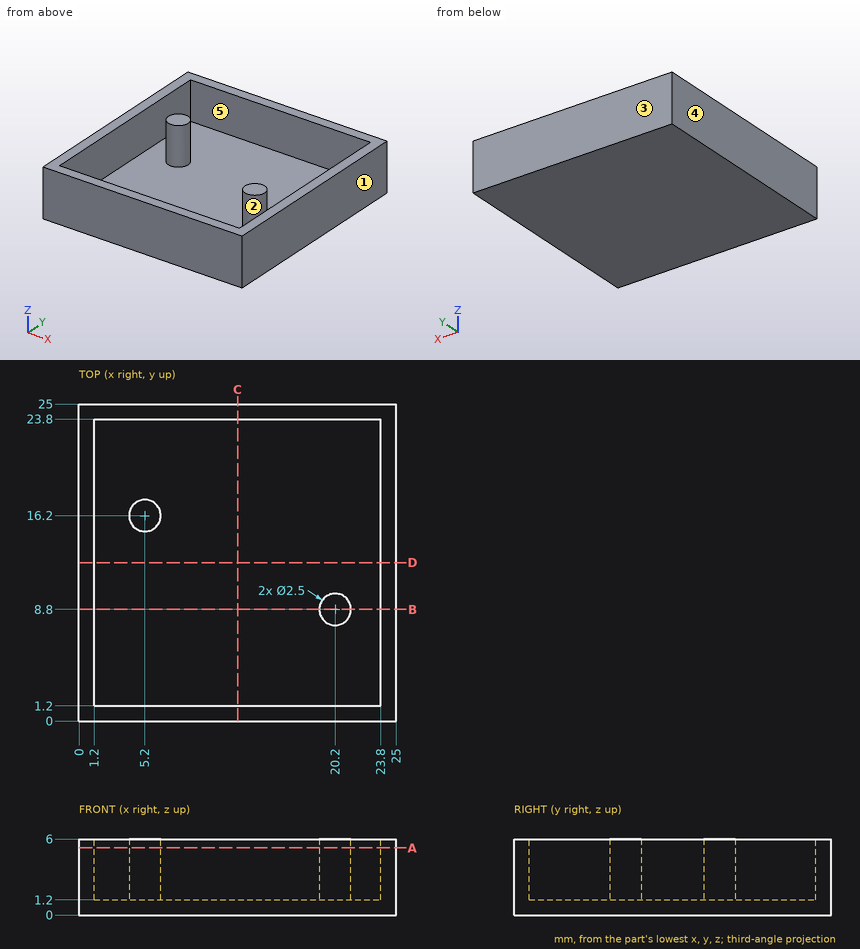
Geometry check sheet. Reference: drawing and pictorial views, mm from the part's lowest x, y, z. A direction names the side the tool comes from. Round coordinates to 2 decimals unless told otherwise and drop trailing zeros. Loops run counter-clockwise (first coordinate to the right, second up) from the corner with the lowest first, then second, coordinate; pieces in that order, holes last. Notation, with made-up numbers: (-30.5, -26.75) - (-1.5, -26.75) arc R13 cw to (-1.5, -5.75) - close; hole circle Ø3 at (9, -25). An arc over 180 degrees is marked (long way). Answer in a Markdown table with one row per item. Add a question column.
Q1. Section check A-A on z = 5.3. Enter the section's corners in (x, y), plus the area to 3 significant figures.
Q2. Section check B-B on y = 8.8. Enter the section's corners in (x, z).
Q3. Section check C-C on x = 12.5. Enter the section's corners in (y, z).
Q4. Gauge pin test, flat ends, axial feed: pin 1 (12 mm diameter, centred on x = 18, y = 13, fed in from -Z); pin 2 (1.5 mm diameter, centred on x = 9.5, y = 12, fed in from +Z). Record the tip position at first contact, or that the pin passes through.
Q5. Tool access check on the marked faces 4 and 5. Record the directions out of +Z, -Z, +X, -X, +Y, -Y that give a thin tool (end or side, any length) a straight path to the whole face; none if there is none.
Q6. Release check for a two-part mould opening along X. For the marked faces 1, 2 and 3 record: pulls with the +X half, pulls with the -X half, needs draft (parallel to the pull), parting line crosses it, or undercut.
Q7. Material ranges on line 1 (Y direction, x = 21.5, z = 1.75); line 2 (Y direction, x = 20.75, z = 1.5), recorded low to high.
Found:
| question | item | result |
|---|---|---|
| 1 | outline | (0, 0) - (25, 0) - (25, 25) - (0, 25) - close; circle Ø2.5 at (5.2, 16.2); circle Ø2.5 at (20.2, 8.8); hole (1.2, 1.2) - (23.8, 1.2) - (23.8, 23.8) - (1.2, 23.8) - close |
| 1 | area | 124 mm² |
| 2 | outline | (0, 0) - (25, 0) - (25, 6) - (23.8, 6) - (23.8, 1.2) - (21.45, 1.2) - (21.45, 6) - (18.95, 6) - (18.95, 1.2) - (1.2, 1.2) - (1.2, 6) - (0, 6) - close |
| 3 | outline | (0, 0) - (25, 0) - (25, 6) - (23.8, 6) - (23.8, 1.2) - (1.2, 1.2) - (1.2, 6) - (0, 6) - close |
| 4 | pin 1 | stops at z = 0 |
| 4 | pin 2 | stops at z = 1.2 |
| 5 | face 4 | +Z, -Z, -X, +Y, -Y |
| 5 | face 5 | +Z |
| 6 | face 1 | pulls with the +X half |
| 6 | face 2 | undercut |
| 6 | face 3 | needs draft |
| 7 | line 1 | y = 0 to 1.2, 23.8 to 25 |
| 7 | line 2 | y = 0 to 1.2, 7.68 to 9.92, 23.8 to 25 |
